from build123d import *

# Parameters (mm, degrees)
F0_R     = 7.9375
F1_DEPTH = 9.525
F2_R     = 1.5875
F3_DEPTH = 25.4
F4_R     = 9.525
F5_R     = 3.175


with BuildPart() as f1:
    # F0 (on Right) → F1 (new body, symmetric)
    with BuildSketch(Plane.YZ):
        with BuildLine():
            Line((431.8, -19.05), (431.8, 19.05))
            Line((431.8, 19.05), (-47.09286, 19.05))
            ThreePointArc((-47.09286, 19.05), (-50.8, 0), (-47.09286, -19.05))
            Line((-47.09286, -19.05), (431.8, -19.05))
        make_face()
        Circle(F0_R, mode=Mode.SUBTRACT)
    extrude(amount=F1_DEPTH, both=True)

    # F2 (on face) → F3 (cut)
    with BuildSketch(Plane.XY.offset(19.05)):
        with Locations((0, 396.875)):
            Circle(F2_R)
        with Locations((0, 314.325)):
            Circle(F2_R)
    extrude(amount=-F3_DEPTH, mode=Mode.SUBTRACT)

    # F4
    f4_edges = [f1.edges().sort_by_distance(p)[0] for p in [
        (0, 431.8, -19.05),
    ]]
    fillet(f4_edges, radius=F4_R)

    # F5
    f5_edges = [f1.edges().sort_by_distance(p)[0] for p in [
        (0, 431.8, 19.05),
        (0, -47.09286, -19.05),
        (0, -47.09286, 19.05),
    ]]
    fillet(f5_edges, radius=F5_R)


solid = f1.part
Here's how the part is built. I have some questions about the finished solid (model axes, mm). Give positions to 0.01 mm unless a question says otherwise; leave off trailing zeros. Order: outer loops, then holes, each group sorted by start corner. A loop starts at its lowest first (then second) coordinate and runs counter-clockwise, first axis right, second up. Notation, with made-up numbers: M 85,25.25 L 114,25.25 A17 cw 114,43.25 Z; hole C 22.5,60.25 d9. An arc over 180 degrees is marked long. Answer as a JSON object with one key per item and string values. Group by question number.
1) We'd pull the mould along Z, two halves only. Please class faces 1 (the flat face through (0, 195, 19.05)), 2 (the cylindrical face through (-0.13, -1.72, -7.75)), 3 (the flat face through (9.525, 187, 0)): pulls with the +Z half, pulls with the -Z half, needs draft (parallel to the pull), parting line crosses it, or undercut.
2) Suppose I cut it at B-B, the plane z = 0. Write out the boundary of the cut face in (x, y) (1 decimal), plus the area to 3 significant figures.
3) Please list where these lines run through material, in increasing order: L1, parallel to Y at x = 0, z = 7; L2, parallel to Y at x = 0, z = 2; L3, parallel to Y at x = 8, z = 1. Write a range as [from, to].
4) I'm going to push flat-ended pins straight in: pin 1 Ø1 at (x, y) = (0, 397.5) entering from +Z; pin 2 Ø2 at (x, z) = (5, -5) entering from -Y; pin 3 Ø12.5 at (y, z) = (0, 0) entering from -X. Where does each tip first touch, or does it pass through?
Results found:
{
 "1": {"face 1": "pulls with the +Z half", "face 2": "undercut", "face 3": "needs draft"},
 "2": {"outline": "M -9.5,-50.8 L 9.5,-50.8 L 9.5,-7.9 L -9.5,-7.9 Z; M -9.5,7.9 L 9.5,7.9 L 9.5,431.8 L -9.5,431.8 Z; hole C 0,314.3 d3.2; hole C 0,396.9 d3.2", "area": "8,880 mm²"},
 "3": {"L1": "[-50.32, -3.74], [3.74, 312.74], [315.91, 395.29], [398.46, 431.8]", "L2": "[-50.76, -7.68], [7.68, 312.74], [315.91, 395.29], [398.46, 431.8]", "L3": "[-50.79, -7.87], [7.87, 431.8]"},
 "4": {"pin 1": "z = -6.35", "pin 2": "y = -50.64", "pin 3": "through"}
}
